Geometry: final body of the model. Coordinates: model frame, mm. Coordinates: 2 decimals unless noted, no trailing zeros. Write each loop counter-clockwise with the first axis right and the second up, starting at its lowest first coordinate (ties: lowest second). Pieces come first, ordered by that corner, then holes. Notation, with made-up numbers: (39, 62) - (61, 62) arc R34 cw to (61, 92) - close; hole circle Ø8 at (2, 19). An arc over 180 degrees is marked (long way). Put each result on its own line as item: value.
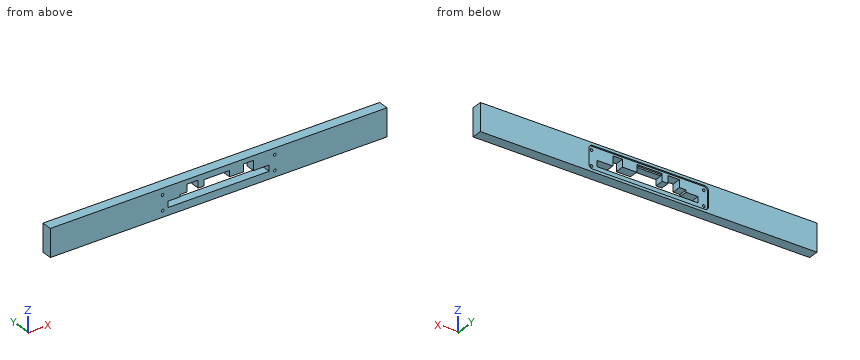
```python
from build123d import *

# Parameters (mm, degrees)
SKETCH008_W          = 450
SKETCH008_H          = 14
PAD008_DEPTH         = 37
SKETCH015_R          = 1.75
POCKET007_DEPTH      = 14.001
POCKET007_DEPTH_BACK = 0.001
SKETCH016_W          = 34
SKETCH016_H          = 2
POCKET008_DEPTH      = 4.5
POCKET010_DEPTH      = 2


with BuildPart() as part:
    # Sketch008 → Pad008 (new body)
    with BuildSketch(Plane.XY):
        with Locations((0, 43)):
            Rectangle(SKETCH008_W, SKETCH008_H)
    extrude(amount=PAD008_DEPTH)

    # Sketch015 (on Face1 of Pad008) → Pocket007 (cut, two sides)
    with BuildSketch(Plane(origin=(0, 50, 0), x_dir=(-1, 0, 0), z_dir=(0, 1, 0))) as pocket007_sk:
        with Locations((-75, 28.5)):
            Circle(SKETCH015_R)
        with Locations((-75, 8.5)):
            Circle(SKETCH015_R)
        with Locations((75, 28.5)):
            Circle(SKETCH015_R)
        with Locations((75, 8.5)):
            Circle(SKETCH015_R)
        Polygon((-67.5, 18), (-46.5, 18), (-46.5, 31), (-33.5, 31), (-33.5, 21), (-14.5, 21), (-14.5, 29), (19.5, 29), (19.5, 21), (27.5, 21), (27.5, 31), (42.5, 31), (42.5, 21), (51.5, 21), (51.5, 18), (67.5, 18), (67.5, 10), (-67.5, 10), align=None)
    extrude(amount=-POCKET007_DEPTH, mode=Mode.SUBTRACT)
    extrude(pocket007_sk.sketch, amount=POCKET007_DEPTH_BACK, mode=Mode.SUBTRACT)

    # Sketch016 (on Face1 of Pocket007) → Pocket008 (cut)
    with BuildSketch(Plane(origin=(0, 50, 0), x_dir=(-1, 0, 0), z_dir=(0, 1, 0))):
        with Locations((2.5, 30)):
            Rectangle(SKETCH016_W, SKETCH016_H)
    extrude(amount=-POCKET008_DEPTH, mode=Mode.SUBTRACT)

    # Sketch019 (on Face1 of Pocket008) → Pocket010 (cut)
    with BuildSketch(Plane(origin=(0, 50, 0), x_dir=(-1, 0, 0), z_dir=(0, 1, 0))):
        with BuildLine():
            ThreePointArc((-75, 33.5), (-78.535534, 32.035534), (-80, 28.5))
            Line((-80, 8.5), (-80, 28.5))
            ThreePointArc((-80, 8.5), (-78.535534, 4.964466), (-75, 3.5))
            Line((75, 3.5), (-75, 3.5))
            ThreePointArc((75, 3.5), (78.535534, 4.964466), (80, 8.5))
            Line((80, 28.500023), (80, 8.5))
            ThreePointArc((80, 28.500023), (78.535526, 32.035542), (75, 33.5))
            Line((-75, 33.5), (75, 33.5))
        make_face()
    extrude(amount=-POCKET010_DEPTH, mode=Mode.SUBTRACT)


solid = part.part
```
1. Section query B-B (x = 38). Return loops of the section in (y, z), then the cut area to 3 significant figures.
Answer below:
outline: (36, 0) - (50, 0) - (50, 3.5) - (48, 3.5) - (48, 10) - (36, 10) - close; (36, 31) - (48, 31) - (48, 33.5) - (50, 33.5) - (50, 37) - (36, 37) - close
area: 206 mm²
2. Ray query, probe 1 along X at (y, z) = (47.25, 23); probe 2 along Z at (x, y) = (75, 41.5); probe 3 along X at (y, z) = (37.25, 12). Return the intervals inside material, ascending. Write a range as from..to.
Answer below:
probe 1: x = -225..-42.5, -27.5..-19.5, 14.5..33.5, 46.5..225
probe 2: z = 0..6.75, 10.25..26.75, 30.25..37
probe 3: x = -225..-67.5, 67.5..225
3. Pin query (flat end, axial travel): pin 1 Ø2 at (x, z) = (-2, 6) entering from +Y; pin 2 Ø1.6 at (x, z) = (-6.5, 29.5) entering from +Y. Return the tip coordinate at first contact, or that it passes through.
Answer below:
pin 1: stops at y = 48
pin 2: stops at y = 45.5
4. Section query C-C (x = -59). Return loops of the section in (y, z), then the cut area to 3 significant figures.
Answer below:
outline: (36, 0) - (50, 0) - (50, 3.5) - (48, 3.5) - (48, 10) - (36, 10) - close; (36, 18) - (48, 18) - (48, 33.5) - (50, 33.5) - (50, 37) - (36, 37) - close
area: 362 mm²
5. Section query A-A (y = 41.5). Return loops of the section in (x, z), then the cut area to 3 significant figures.
Answer below:
outline: (-225, 0) - (225, 0) - (225, 37) - (-225, 37) - close; hole circle Ø3.5 at (-75, 8.5); hole circle Ø3.5 at (-75, 28.5); hole (-67.5, 10) - (67.5, 10) - (67.5, 18) - (46.5, 18) - (46.5, 31) - (33.5, 31) - (33.5, 21) - (14.5, 21) - (14.5, 29) - (-19.5, 29) - (-19.5, 21) - (-27.5, 21) - (-27.5, 31) - (-42.5, 31) - (-42.5, 21) - (-51.5, 21) - (-51.5, 18) - (-67.5, 18) - close; hole circle Ø3.5 at (75, 8.5); hole circle Ø3.5 at (75, 28.5)
area: 14,700 mm²
